Autodesk Inventor part; units mm, degrees
ref_plane "YZ Plane" through (0, 0, 0) normal (1, 0, 0) x (0, 1, 0)
ref_plane "XZ Plane" through (0, 0, 0) normal (0, 1, 0) x (-1, 0, 0)
ref_plane "XY Plane" through (0, 0, 0) normal (0, 0, 1) x (1, 0, 0)
sketch "Sketch1" plane through (0, 0, 0) normal (0, 1, 0) x (-1, 0, 0)
  line L0 (0, 0) -> (28.575, 0)
  line L1 (28.575, 0) -> (0, 0)
  line L2 (0, 0) -> (-14.2875, -24.7467)
  line L3 (0, 0) -> (28.575, 0) construction
  line L4 (0, 0) -> (-14.2875, 24.7467)
  line L5 (0, 0) -> (28.575, 0) construction
  circle A0 centre (28.575, 0) radius 2.54
  circle A1 centre (-14.2875, -24.7467) radius 2.54
  circle A2 centre (-14.2875, 24.7467) radius 2.54
  circle A3 centre (0, 0) radius 3.175
  dimension "d0" = 28.575
  dimension "d1" = 28.575
  dimension "d2" = 120
  dimension "d3" = 28.575
  dimension "d4" = 120
  dimension "d5" = 5.08
  dimension "d6" = 5.08
  dimension "d7" = 5.08
  dimension "d9" = 6.35
sketch "Sketch2" plane through (0, 0, 0) normal (0, 1, 0) x (-1, 0, 0)
  circle A0 centre (28.575, 0) radius 2.54
  circle A1 centre (-14.2875, -24.7467) radius 2.54
  circle A2 centre (-14.2875, 24.7467) radius 2.54
  circle A3 centre (28.575, 0) radius 4.445
  circle A4 centre (-14.2875, -24.7467) radius 4.445
  circle A5 centre (-14.2875, 24.7467) radius 4.445
  circle A6 centre (0, 0) radius 6.35
  circle A7 centre (0, 0) radius 9.525
  line L0 (28.575, 4.445) -> (28.575, -4.445)
  line L1 (-14.2875, 24.7467) -> (0, 0)
  line L2 (0, 0) -> (-14.2875, 24.7467)
  line L3 (-14.2875, 24.7467) -> (-10.438, 26.9692)
  line L4 (-14.2875, 24.7467) -> (-18.137, 22.5242)
  line L5 (0, 0) -> (-14.2875, -24.7467)
  line L6 (-10.438, -26.9692) -> (-14.2875, -24.7467)
  line L7 (-18.137, -22.5242) -> (-14.2875, -24.7467)
  arc A8 (4.7625, 8.2489) -> (28.575, 4.445) centre (26.9969, 71.0017) ccw
  arc A9 (28.575, -4.445) -> (4.7625, -8.2489) centre (26.881, -70.2762) ccw
  arc A10 (4.7625, -8.2489) -> (-10.438, -26.9692) centre (47.4204, -58.4177) ccw
  arc A11 (-18.137, -22.5242) -> (-9.525, 0) centre (-74.3014, 11.8584) ccw
  arc A12 (-9.525, 0) -> (-18.137, 22.5242) centre (-78.365, -13.4121) ccw
  arc A13 (-10.438, 26.9692) -> (4.7625, 8.2489) centre (47.4204, 58.4177) ccw
  arc A14 (-3.702, 16.9073) -> (16.4951, 5.2598) centre (24.8224, 43.0343) ccw
  arc A15 (16.4931, -5.2477) -> (-3.702, -16.9073) centre (24.8816, -43.0963) ccw
  line L8 (-9.525, 0) -> (-10.9982, 0)
  arc A16 (-12.7912, -11.6596) -> (-12.8557, 11.635) centre (-49.0728, -0.1126) ccw
  dimension "d10" = 8.89
  dimension "d11" = 8.89
  dimension "d12" = 8.89
  dimension "d13" = 12.7
  dimension "d14" = 19.05
  dimension "d15" = 1.4732
extrude "Extrusion1" add sketch "Sketch2" along normal blind 12.7 contours A0 L0 A3 | A0 L0 A9 A7 A8 | L6 A1 L5 A4 | A11 A7 L5 A4 | L4 A2 L1 A5 | A13 A7 L1 A5 | A8 A13 A14 | A15 A10 A9 | A7 L5 A6 L1 | A4 L7 A1 L6 | A10 A4 L5 A7 | L1 A6 L5 A7 | A5 L3 A2 L4 | A7 A12 A5 L1 | A5 L1 A2 L3 | L8 A16 A12 | A11 A16 L8 | L1 L5 A6 | A6 L5 L1 | L5 A1 L7 A4
hole "Hole1" at (0, 0, 0) direction (0, 1, 0) diameter 6.35 end through all
sketch "Sketch3" plane through (0, 12.7, 0) normal (0, 1, 0) x (1, 0, 0)
  circle A0 centre (0, 0) radius 3.175
hole "Hole2" at (0, 12.7, 0) direction (0, -1, 0) diameter 6.604 end through all
sketch "Sketch4" plane through (0, 12.7, 0) normal (0, 1, 0) x (1, 0, 0)
  circle A0 centre (-10.3993, 5.2212) radius 3.175
  circle A1 centre (-10.8149, -4.2948) radius 3.175
  point P0 (0, 0)
hole "Hole3" at (-10.3993, 12.7, -5.2212) at (-10.8149, 12.7, 4.2948) direction (0, -1, 0) diameter 6.35 depth 162.56
sketch "Sketch5" plane through (0, 12.7, 0) normal (0, 1, 0) x (1, 0, 0)
  arc A0 (-16.4951, -5.2598) -> (-28.575, -4.445) centre (-26.9969, -71.0017) ccw
  arc A1 (-28.575, 4.445) -> (-16.4931, 5.2477) centre (-26.881, 70.2762) ccw
  line L0 (-16.4951, -5.2598) -> (-16.4931, 5.2477)
  arc A2 (10.438, -26.9692) -> (3.702, -16.9073) centre (-47.4204, -58.4177) ccw
  arc A3 (12.8557, -11.635) -> (18.137, -22.5242) centre (78.365, 13.4121) ccw
  line L1 (3.702, -16.9073) -> (12.8557, -11.635)
  arc A4 (18.137, 22.5242) -> (12.7912, 11.6596) centre (74.3014, -11.8584) ccw
  arc A5 (3.702, 16.9073) -> (10.438, 26.9692) centre (-47.4204, 58.4177) ccw
  line L2 (12.7912, 11.6596) -> (3.702, 16.9073)
  arc A6 (18.137, 22.5242) -> (10.438, 26.9692) centre (14.2875, 24.7467) ccw
  arc A7 (-28.575, 4.445) -> (-28.575, -4.445) centre (-28.575, 0) ccw
  point P0 (0, 0)
sketch "Sketch6" plane through (0, 12.7, 0) normal (0, 1, 0) x (1, 0, 0)
  arc A0 (-13.4646, 6.0485) -> (-8.668, 7.8826) centre (-10.3993, 5.2212) ccw
  line L0 (-10.3993, 5.2212) -> (-7.2243, 5.2212)
  line L1 (-10.3993, 5.2212) -> (-13.5743, 5.2212)
  line L2 (-13.5743, 5.2212) -> (-13.5743, 8.7596)
  line L3 (-13.5743, 8.7596) -> (-7.2855, 8.8652)
  line L4 (-7.2855, 8.8652) -> (-7.2243, 5.2212)
  arc A1 (-9.9167, -7.3401) -> (-13.4529, -6.0614) centre (-10.8149, -4.2948) ccw
  line L5 (-10.8149, -4.2948) -> (-13.9899, -4.2948)
  line L6 (-13.9899, -4.2948) -> (-13.9899, -9.3241)
  line L7 (-10.8149, -4.2948) -> (-7.6399, -4.2948)
  line L8 (-7.6399, -4.2948) -> (-7.6399, -9.0772)
  line L9 (-7.6399, -9.0772) -> (-13.9899, -9.3241)
  point P0 (0, 0)
extrude "Extrusion2" cut sketch "Sketch6" against normal blind 25.4 contours L2 L3 L4 L0 L1 | L8 L9 L6 L5 L7
sketch "Sketch7" plane through (0, 12.7, 0) normal (0, 1, 0) x (1, 0, 0)
  arc A0 (12.7912, 11.6596) -> (12.8557, -11.635) centre (49.0728, 0.1126) ccw
  arc A1 (12.7912, 11.6596) -> (12.8557, -11.635) centre (49.0728, 0.1126) ccw
  arc A2 (-7.2803, 8.5554) -> (3.702, 16.9073) centre (-24.8816, 43.0963) ccw
  arc A3 (-16.4931, 5.2477) -> (3.702, 16.9073) centre (-24.8816, 43.0963) ccw
  arc A4 (-13.9899, -5.9006) -> (-16.4951, -5.2598) centre (-24.8224, -43.0343) ccw
  arc A5 (3.702, -16.9073) -> (-16.4951, -5.2598) centre (-24.8224, -43.0343) ccw
  arc A6 (-28.575, 4.445) -> (-16.4931, 5.2477) centre (-26.881, 70.2762) ccw
  line L0 (-16.4931, 5.2477) -> (-16.4951, -5.2598)
  line L1 (3.702, -16.9073) -> (12.8557, -11.635)
  line L2 (3.702, 16.9073) -> (12.7912, 11.6596)
  point P0 (0, 0)
  point P1 (-7.2803, 8.5554)
  point P2 (-13.9899, -5.9006)
extrude "Extrusion3" cut sketch "Sketch7" against normal blind 25.4
extrude "Extrusion4" cut sketch "Sketch5" against normal blind 25.4
sketch "Sketch9" plane through (3.702, 0, 16.9073) normal (-0.4991072, 0, -0.8665403) x (-0.8665403, 0, 0.4991072)
  line L0 (0, 0) -> (0, 12.7)
  line L1 (0, 6.35) -> (-10.5635, 6.35)
  line L2 (-10.5635, 0) -> (-10.5635, 12.7)
  line L3 (-7.8001, 12.7) -> (-2.7201, 12.7)
  line L4 (-5.2601, 12.7) -> (-5.2307, 0)
  circle A0 centre (-5.2454, 6.35) radius 1.0065
  dimension "d45" = 2.013
extrude "Extrusion5" add sketch "Sketch9" along normal blind 7.5946
thread "Thread1"
properties part number "screw in stablity"
The listing builds one solid part. Answer for the finished solid, in the listing's coordinates (mm). Round coordinates to 2 decimals unless told otherwise and drop trailing zeros. Write each loop counter-clockwise with the first axis right and the second up, starting at its lowest first coordinate (ties: lowest second). Pieces come first, ordered by that corner, then holes. Notation, with made-up numbers: (41.25, -12.75) - (47.25, -12.75) arc R25 cw to (47.25, 21.25) - close; hole circle Ø8 at (38, 53.5). An arc over 180 degrees is marked (long way). Use a Markdown table: item, result. Add a question column.
1. For a pull along Z with two mould halves and no side action, classify faces 1 (the face through (6.568, 7.333, 10.936)), 2 (the face through (16.59, 6.26, 28.55)), 3 (the face through (4.47, 6.36, 7.7)) as +Z half, -Z half, draft (parallel to the pull), parting line (faces both ways), or undercut.
2. The part is cut by section B-B (z = 23). Write down the section's boundary in (x, y), and give its area (3 significant figures).
3. The part is cut by section D-D (x = 10). Write down the section's boundary in (y, z).
4. Consider line 1 (X direction, y = 9.75, z = 25); line 2 (Z direction, x = 12.75, y = 6.25); line 3 (X direction, y = 11.25, z = 25.75). Determine where each line is inside the solid, lowest interval first.
5. The part is cut by section A-A (x = 12). Write down the section's boundary in (y, z), and give its area (3 significant figures).
6. Flat-ended cylindrical pins translate along their axes: P1, Ø1, axis at x = 8.5, z = 12.5, coming from the -Y side; P2, Ø1.5, axis at x = 6.5, y = 7.5, coming from the +Z side; P3, Ø1, axis at x = 11, y = 6.5, coming from the +Z side. Find the tip coordinate at first contact, or state that the pin passes through.
7. The part is cut by section C-C (y = 8.5). Write down the section's boundary in (x, z) (1 decimal).
Reported:
| question | item | result |
|---|---|---|
| 1 | face 1 | undercut |
| 1 | face 2 | parting line |
| 1 | face 3 | -Z half |
| 2 | outline | (8.1, 0) - (12.44, 0) - (12.44, 12.7) - (8.1, 12.7) - close; (16.13, 0) - (18.37, 0) - (18.37, 12.7) - (16.13, 12.7) - close |
| 2 | area | 83.7 mm^2 |
| 3 | outline | (0, 13.28) - (12.7, 13.28) - (12.7, 26.18) - (0, 26.18) - close |
| 4 | line 1 | 9.32 to 11.76, 16.81 to 18.73 |
| 4 | line 2 | 11.7 to 22.72, 26.77 to 28.92 |
| 4 | line 3 | 9.76 to 11.95, 16.62 to 18.62 |
| 5 | outline | (0, 12.13) - (12.7, 12.13) - (12.7, 23.64) - (0, 23.64) - close; (0, 25.85) - (12.7, 25.85) - (12.7, 28.56) - (0, 28.56) - close |
| 5 | area | 181 mm^2 |
| 6 | P1 | y = 5.55 |
| 6 | P2 | z = 21.71 |
| 6 | P3 | z = 28.21 |
| 7 | outline | (3.7, 16.9) - (12.9, 11.6) arc R70.1 cw to (18.1, 22.5) arc R4.4 ccw to (10.4, 27) arc R65.9 cw to start; hole circle Ø5.1 at (14.3, 24.7) |
